CAD build for the part. Positions are in the model's coordinates, mm. Coordinates: 2 decimals unless noted, no trailing zeros. Answer in a Markdown table with one row per item. Add a question column.
Q1. Band-saw the part on A-A (z = 1.5). State how many separate pieces and enclosed holes the cut face has, and give its area (3 significant figures).
Q2. Pin check, flat tip, straight feed: pin 1 (11 mm diameter, centred on x = 90.76, y = -48.27, fed in from -Z). Stop position of the tip, or through.
Q3. Drill centre lines: line 1 along Y through (x, z) = (-84, 3.55); line 2 along Y through (x, z) = (140, 4.05). Where is each one in solid material? Low to high. Write a range as from..to.
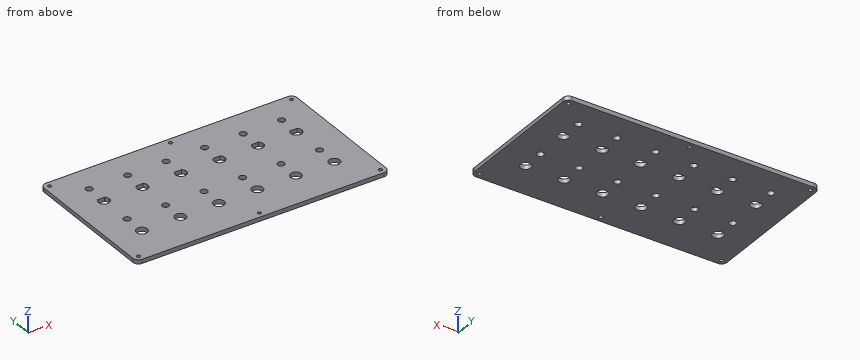
```python
from build123d import *

# Parameters (mm, degrees)
F0_R     = 6.25
F1_DEPTH = 4.7625
F2_D     = 8
F4_D     = 4.1656


# Not quite as in the source:
# - a feature names something its author has since deleted; it is built from what else it names


with BuildPart() as f1:
    # F0 (on Top) → F1 (new body)
    with BuildSketch(Plane.XY):
        with BuildLine():
            Line((163.7876496315, 73.9668203354), (-115.6123503685, 73.9668203354))
            ThreePointArc((-115.6123503685, 73.9668203354), (-120.102478429, 72.1069483959), (-121.9623503685, 67.6168203354))
            Line((-121.9623503685, 67.6168203354), (-121.9623503685, -84.7831796646))
            ThreePointArc((-121.9623503685, -84.7831796646), (-120.102478429, -89.2733077251), (-115.6123503685, -91.1331796646))
            Line((-115.6123503685, -91.1331796646), (163.7876496315, -91.1331796646))
            ThreePointArc((163.7876496315, -91.1331796646), (168.277777692, -89.2733077251), (170.1376496315, -84.7831796646))
            Line((170.1376496315, -84.7831796646), (170.1376496315, 67.6168203354))
            ThreePointArc((170.1376496315, 67.6168203354), (168.277777692, 72.1069483959), (163.7876496315, 73.9668203354))
        make_face()
        with Locations((-87.0373503685, -48.2706796646)):
            Circle(F0_R, mode=Mode.SUBTRACT)
        with Locations((-42.5873503685, -48.2706796646)):
            Circle(F0_R, mode=Mode.SUBTRACT)
        with Locations((1.8626496315, -48.2706796646)):
            Circle(F0_R, mode=Mode.SUBTRACT)
        with Locations((46.3126496315, -48.2706796646)):
            Circle(F0_R, mode=Mode.SUBTRACT)
        with Locations((90.7626496315, -48.2706796646)):
            Circle(F0_R, mode=Mode.SUBTRACT)
        with Locations((135.2126496315, -48.2706796646)):
            Circle(F0_R, mode=Mode.SUBTRACT)
        with BuildLine():
            ThreePointArc((-83.0950236494, 21.6666203354), (-81.3936794889, 19.5022400424), (-80.7873503685, 16.8168203354))
            ThreePointArc((-80.7873503685, 16.8168203354), (-89.7227700755, 11.1731494558), (-90.9796770876, 21.6666203354))
            ThreePointArc((-90.9796770876, 21.6666203354), (-87.0373503685, 23.0668203354), (-83.0950236494, 21.6666203354))
        make_face(mode=Mode.SUBTRACT)
        with BuildLine():
            ThreePointArc((-38.6450236494, 21.6666203354), (-36.9436794889, 19.5022400424), (-36.3373503685, 16.8168203354))
            ThreePointArc((-36.3373503685, 16.8168203354), (-45.2727700755, 11.1731494558), (-46.5296770876, 21.6666203354))
            ThreePointArc((-46.5296770876, 21.6666203354), (-42.5873503685, 23.0668203354), (-38.6450236494, 21.6666203354))
        make_face(mode=Mode.SUBTRACT)
        with BuildLine():
            ThreePointArc((5.8049763506, 21.6666203354), (7.5063205111, 19.5022400424), (8.1126496315, 16.8168203354))
            ThreePointArc((8.1126496315, 16.8168203354), (-0.8227700755, 11.1731494558), (-2.0796770876, 21.6666203354))
            ThreePointArc((-2.0796770876, 21.6666203354), (1.8626496315, 23.0668203354), (5.8049763506, 21.6666203354))
        make_face(mode=Mode.SUBTRACT)
        with BuildLine():
            ThreePointArc((50.2549763506, 21.6666203354), (51.9563205111, 19.5022400424), (52.5626496315, 16.8168203354))
            ThreePointArc((52.5626496315, 16.8168203354), (43.6272299245, 11.1731494558), (42.3703229124, 21.6666203354))
            ThreePointArc((42.3703229124, 21.6666203354), (46.3126496315, 23.0668203354), (50.2549763506, 21.6666203354))
        make_face(mode=Mode.SUBTRACT)
        with BuildLine():
            ThreePointArc((94.7049763506, 21.6666203354), (96.4063205111, 19.5022400424), (97.0126496315, 16.8168203354))
            ThreePointArc((97.0126496315, 16.8168203354), (88.0772299245, 11.1731494558), (86.8203229124, 21.6666203354))
            ThreePointArc((86.8203229124, 21.6666203354), (90.7626496315, 23.0668203354), (94.7049763506, 21.6666203354))
        make_face(mode=Mode.SUBTRACT)
        with BuildLine():
            ThreePointArc((139.1549763506, 21.6666203354), (140.8563205111, 19.5022400424), (141.4626496315, 16.8168203354))
            ThreePointArc((141.4626496315, 16.8168203354), (132.5272299245, 11.1731494558), (131.2703229124, 21.6666203354))
            ThreePointArc((131.2703229124, 21.6666203354), (135.2126496315, 23.0668203354), (139.1549763506, 21.6666203354))
        make_face(mode=Mode.SUBTRACT)
        with BuildLine():
            Line((-46.5296770876, 21.6666203354), (-38.6450236494, 21.6666203354))
            ThreePointArc((-38.6450236494, 21.6666203354), (-42.5873503685, 23.0668203354), (-46.5296770876, 21.6666203354))
        make_face()
        with BuildLine():
            Line((-90.9796770876, 21.6666203354), (-83.0950236494, 21.6666203354))
            ThreePointArc((-83.0950236494, 21.6666203354), (-87.0373503685, 23.0668203354), (-90.9796770876, 21.6666203354))
        make_face()
        with BuildLine():
            Line((131.2703229124, 21.6666203354), (139.1549763506, 21.6666203354))
            ThreePointArc((139.1549763506, 21.6666203354), (135.2126496315, 23.0668203354), (131.2703229124, 21.6666203354))
        make_face()
        with BuildLine():
            Line((42.3703229124, 21.6666203354), (50.2549763506, 21.6666203354))
            ThreePointArc((50.2549763506, 21.6666203354), (46.3126496315, 23.0668203354), (42.3703229124, 21.6666203354))
        make_face()
        with BuildLine():
            Line((-2.0796770876, 21.6666203354), (5.8049763506, 21.6666203354))
            ThreePointArc((5.8049763506, 21.6666203354), (1.8626496315, 23.0668203354), (-2.0796770876, 21.6666203354))
        make_face()
        with BuildLine():
            Line((86.8203229124, 21.6666203354), (94.7049763506, 21.6666203354))
            ThreePointArc((94.7049763506, 21.6666203354), (90.7626496315, 23.0668203354), (86.8203229124, 21.6666203354))
        make_face()
    extrude(amount=F1_DEPTH)

    # F2 (through all)
    with Locations(Plane(origin=(0, 0, 0), x_dir=(1, 0, 0), z_dir=(0, 0, -1))):
        with Locations((46.3126496315, -42.2168203354), (135.2126496315, -42.2168203354), (-87.0373503685, -42.2168203354), (-42.5873503685, -42.2168203354), (1.8626496315, -42.2168203354), (90.7626496315, -42.2168203354), (1.8626496315, 22.8706796646), (-87.0373503685, 22.8706796646), (90.7626496315, 22.8706796646), (-42.5873503685, 22.8706796646), (135.2126496315, 22.8706796646), (46.3126496315, 22.8706796646)):
            Hole(F2_D / 2)

    # F4 (through all)
    with Locations(Plane.XY.offset(4.7625)):
        with Locations((-115.6123503685, 67.6168203354), (163.7876496315, 67.6168203354), (163.7876496315, -84.7831796646), (-115.6123503685, -84.7831796646), (24.0876496315, 67.6168203354), (24.0876496315, -84.7831796646)):
            Hole(F4_D / 2)


solid = f1.part
```
Checked values:
| question | item | result |
|---|---|---|
| 1 | separate pieces | 1 |
| 1 | enclosed holes | 30 |
| 1 | area | 46,100 mm² |
| 2 | pin 1 | passes through |
| 3 | line 1 | y = -91.13..-53.73, -42.81..-25.47, -20.27..11.35, 21.67..39.61, 44.82..73.97 |
| 3 | line 2 | y = -91.13..-52.29, -44.25..12.8, 20.83..73.97 |
